from build123d import *

# Parameters (mm, degrees)
BOSS_EXTRUDE1_DEPTH = 166.124


with BuildPart() as part:
    # Sketch1 → Boss-Extrude1 (new body)
    with BuildSketch(Plane(origin=(0, 0, 0), x_dir=(0, 0, -1), z_dir=(1, 0, 0))):
        with BuildLine():
            Line((0, 35), (3.175, 35))
            Line((3.175, 35), (3.175, 63.720329141))
            ThreePointArc((3.175, 63.720329141), (3.559257641, 64.508276695), (4.416722694, 64.690674512))
            Line((4.416722694, 64.690674512), (42.283933187, 55.257575303))
            ThreePointArc((42.283933187, 55.257575303), (42.971366415, 54.656918005), (42.88448418, 53.748179809))
            Line((42.88448418, 53.748179809), (27.463573236, 29.652781316))
            Line((27.463573236, 29.652781316), (30.137792194, 27.941297175))
            Line((30.137792194, 27.941297175), (9.211368438, -4.756545468))
            ThreePointArc((9.211368438, -4.756545468), (3.595870766, -6.860088565), (0, -2.061294853))
            Line((0, -2.061294853), (0, 35))
        make_face()
    extrude(amount=BOSS_EXTRUDE1_DEPTH)


solid = part.part
The listing builds one solid part. Answer for the finished solid, in the listing's coordinates (mm). A direction names the side the tool comes from. Coordinates: 2 decimals unless noted, no trailing zeros. Order: outer loops, then holes, each group sorted by start corner. A loop starts at its lowest first (then second) coordinate and runs counter-clockwise, first axis right, second up. Notation, with made-up numbers: (15.5, -17.5) -> (60.5, -17.5) arc R17 cw to (60.5, -9.5) -> close; hole circle Ø3 at (-35.75, -13.5). An arc over 180 degrees is marked (long way). Answer in a Markdown table with one row per item. Add a question column.
Item 1: Which of the six approach directions +Z, -Z, +X, -X, +Y, -Y give full straight-line access (tool end or side, diameter ignored) to faces 1 (the face through (82, 49, -3.175)), 2 (the face through (82, 16, 0))?
Item 2: Find section C-C (y = 6). Write down the section's boundary in (x, z).
Item 3: Find section B-B (z = -38.5). Write down the section's boundary in (x, y).
Item 4: Each of these flat-tipped pins is pushed along its axis until it touches: P1, Ø3.5, axis at x = 108.5, z = -1, coming from the +Y side; P2, Ø5, axis at x = 51, z = -24, coming from the +Y side; P3, Ø6, axis at y = 47, z = -13.5, coming from the -X side; P4, Ø3, axis at x = 112, z = -28, coming from the +Y side. Where does it stop, or does it pass through?
Item 5: Find the intervals of material crossed by L1, parallel to Y at x = 126, z = -34; L2, parallel to Y at x = 54, z = -5; L3, parallel to Z at x = 66.5, y = 17.5, in increasing order. Write a range as from..to.
Item 6: Find section A-A (x = 66). Write down the section's boundary in (y, z) (3 decimals).
Result set:
| question | item | result |
|---|---|---|
| 1 | face 1 | +Z, +X, -X, +Y |
| 1 | face 2 | +Z, +X, -X, +Y, -Y |
| 2 | outline | (0, -16.1) -> (166.12, -16.1) -> (166.12, 0) -> (0, 0) -> close |
| 3 | outline | (0, 46.9) -> (166.12, 46.9) -> (166.12, 56.2) -> (0, 56.2) -> close |
| 4 | P1 | stops at y = 35 |
| 4 | P2 | stops at y = 60.44 |
| 4 | P3 | stops at x = 0 |
| 4 | P4 | stops at y = 59.19 |
| 5 | L1 | y = 39.87..57.32 |
| 5 | L2 | y = -7.06..64.55 |
| 5 | L3 | z = -23.46..0 |
| 6 | outline | (-4.757, -9.211) -> (27.941, -30.138) -> (29.653, -27.464) -> (53.748, -42.884) arc R1 ccw to (55.258, -42.284) -> (64.691, -4.417) arc R1 ccw to (63.72, -3.175) -> (35, -3.175) -> (35, 0) -> (-2.061, 0) arc R5 ccw to start |
